Can you work these out from the model? Positions are in its coordinate system, mm. A direction names the side the tool comes from. Give positions to 0.01 mm unless a question says otherwise; leave off trailing zeros. Write each loop counter-clockwise with the first axis right and the second up, starting at its lowest first coordinate (ties: lowest second). Pieces come first, ordered by that corner, then holes. Notation, with made-up numbers: (-0.5, 60) -> (20.5, 60) arc R26 ccw to (20.5, 75) -> close; hole circle Ø5 at (-20.75, 21). An arc over 180 degrees is marked (long way). Answer as CSV lines item,"result". Start each with the question number.
1. If we section it at B-B on z = 11.25: Write out the boundary of the cut face in (x, y).
2. If we section it at C-C on x = -7.25: Write out the boundary of the cut face in (y, z), plus the area to 3 significant figures.
3. I'm going to push flat-ended pins straight in: P1, Ø1.9, axis at x = -1.5, z = 8, coming from the -Y side; P2, Ø3, axis at x = 8.5, z = 10, coming from the -Y side; P3, Ø7.5, axis at x = -4.5, y = -5, coming from the +Z side. Where does each tip first touch, or does it pass through?
4. If we section it at D-D on x = -4.5: Write out the boundary of the cut face in (y, z), plus the area to 3 significant figures.
5. If we mould it in two halves opening along X, with no side actions, what happens to faces 4 (the face through (0, 19.05, 6)), 5 (the face through (-12.7, 4, 5)), 6 (the face through (6.35, 4, 10))? For each: pulls with the +X half, pulls with the -X half, needs draft (parallel to the pull), parting line crosses it, or undercut.
6. If we section it at A-A on y = 1.5: Write out the boundary of the cut face in (x, z).
7. On a 3-axis mill with a long thin cutter (end or side, diameter ignored), from which of +Z, -Z, +X, -X, +Y, -Y can I reach the whole of each face in a straight line? I mean faces 1 (the face through (0, 7.62, 10)), 2 (the face through (9, 0, 9)), 3 (the face through (0, 0, 0)). Say none if no direction works.
8. I need wall thicknesses on line 1 (Z direction, x = 7.75, y = -2.5); line 2 (Y direction, x = 0, z = 8); line 3 (Y direction, x = -10.75, z = 7). Which ranges of each line are inside material? Lowest first, please. Write a range as [from, to].
```python
from build123d import *

# Parameters (mm, degrees)
F0_W     = 25.4
F0_H     = 38.1
F1_DEPTH = 6.35
F2_W     = 25.4
F2_H     = 19.05
F3_DEPTH = 6.35
F4_W     = 12.7
F4_H     = 15.24
F5_DEPTH = 6.35


with BuildPart() as f1:
    # F0 (on Top) → F1 (new body)
    with BuildSketch(Plane.XY):
        Rectangle(F0_W, F0_H)
    extrude(amount=F1_DEPTH)

    # F2 (on face) → F3 (join)
    with BuildSketch(Plane.XY.offset(6.35)):
        with Locations((0, 9.525)):
            Rectangle(F2_W, F2_H)
    extrude(amount=F3_DEPTH)

    # F4 (on face) → F5 (cut, symmetric)
    with BuildSketch(Plane.XY.offset(12.7)):
        Rectangle(F4_W, F4_H)
    extrude(amount=F5_DEPTH, both=True, mode=Mode.SUBTRACT)


solid = f1.part
```
Computed values:
1,outline,"(-12.7, 0) -> (-6.35, 0) -> (-6.35, 7.62) -> (6.35, 7.62) -> (6.35, 0) -> (12.7, 0) -> (12.7, 19.05) -> (-12.7, 19.05) -> close"
2,outline,"(-19.05, 0) -> (19.05, 0) -> (19.05, 12.7) -> (0, 12.7) -> (0, 6.35) -> (-19.05, 6.35) -> close"
2,area,"363 mm2"
3,P1,"stops at y = 7.62"
3,P2,"stops at y = 0"
3,P3,"stops at z = 6.35"
4,outline,"(-19.05, 0) -> (19.05, 0) -> (19.05, 12.7) -> (7.62, 12.7) -> (7.62, 6.35) -> (-19.05, 6.35) -> close"
4,area,"315 mm2"
5,face 4,"needs draft"
5,face 5,"pulls with the -X half"
5,face 6,"undercut"
6,outline,"(-12.7, 0) -> (12.7, 0) -> (12.7, 12.7) -> (6.35, 12.7) -> (6.35, 6.35) -> (-6.35, 6.35) -> (-6.35, 12.7) -> (-12.7, 12.7) -> close"
7,face 1,"+Z, -Y"
7,face 2,"+Z, +X, -X, -Y"
7,face 3,"-Z, +X, -X, +Y, -Y"
8,line 1,"z = [0, 6.35]"
8,line 2,"y = [7.62, 19.05]"
8,line 3,"y = [0, 19.05]"
